Source: CAD feature listing. Evaluate the final solid. Frame: model axes, mm. Round coordinates to 2 decimals unless told otherwise and drop trailing zeros. Order: outer loops, then holes, each group sorted by start corner. A loop starts at its lowest first (then second) coordinate and runs counter-clockwise, first axis right, second up. Notation, with made-up numbers: (77.25, -13) - (127.25, -13) arc R25 ccw to (127.25, 6) - close; hole circle Ø1 at (10, 19.25). An arc over 180 degrees is marked (long way). Return JSON: item names as keys, results as strings. Group by question number.
1) Mould query, pull axis X, two halves, no side actions, for faces 1 (the cylindrical face through (79.297, -123.986, 1.521)), 2 (the cylindrical face through (-83, 99, 2)), 3 (the cylindrical face through (-43.67, 95.48, 1.48)). Classes: pulls with the +X half, pulls with the -X half, needs draft (parallel to the pull), parting line crosses it, or undercut.
2) Contact query for flat-ended pins moving along their axis: P1, Ø6, axis at x = 44, y = 93, coming from the +Z side; P2, Ø1, axis at x = -67.5, z = 1, coming from the -Y side. Output: stop coordinate, or through.
3) Section B-B, the plane x = -70. Return loops of the section in (y, z), plus the area to 3 significant figures.
4) Section A-A, the plane x = -44. Return loops of the section in (y, z).
5) Ray query, line 1 (Y direction, x = 11.5, z = 0.7); line 2 (Y direction, x = -44, z = 0.8); line 3 (Y direction, x = 77, z = 2.35). Return the intervals inside material, ascending. Write a range as from..to.
```python
from build123d import *

# Parameters (mm, degrees)
SKETCH_1_W          = 170
SKETCH_1_H          = 200
EXTRUDE_1_DEPTH     = 3
SKETCH_4_W          = 170
SKETCH_4_H          = 30
EXTRUDE_2_DEPTH     = 3
FILLET_1_R          = 20
FILLET_2_R          = 5
SKETCH_6_R          = 1.5
CUT_EXTRUDE_3_DEPTH = 4
SKETCH_7_R          = 2.5
CUT_EXTRUDE_4_DEPTH = 10


with BuildPart() as part:
    # 草图1 → 凸台-拉伸1 (new body)
    with BuildSketch(Plane.XY):
        Rectangle(SKETCH_1_W, SKETCH_1_H)
    extrude(amount=EXTRUDE_1_DEPTH)

    # 草图4 → 凸台-拉伸2 (add)
    with BuildSketch(Plane(origin=(0, 0, 0), x_dir=(-1, 0, 0), z_dir=(0, 0, -1))):
        with Locations((0, -115)):
            Rectangle(SKETCH_4_W, SKETCH_4_H)
    extrude(amount=-EXTRUDE_2_DEPTH)

    # 圆角1
    fillet_1_edges = [part.edges().sort_by_distance(p)[0] for p in [
        (-85, -130, 1.5),
        (85, -130, 1.5),
    ]]
    fillet(fillet_1_edges, radius=FILLET_1_R)

    # 圆角2
    fillet_2_edges = [part.edges().sort_by_distance(p)[0] for p in [
        (-85, 100, 1.5),
        (85, 100, 1.5),
    ]]
    fillet(fillet_2_edges, radius=FILLET_2_R)

    # 草图6 → 切除-拉伸3 (cut, through all)
    with BuildSketch(Plane.XY.offset(3)):
        with Locations((11.5, 5)):
            Circle(SKETCH_6_R)
        with Locations((11.5, 15)):
            Circle(SKETCH_6_R)
        with Locations((11.5, 65)):
            Circle(SKETCH_6_R)
        with Locations((11.5, 75)):
            Circle(SKETCH_6_R)
    extrude(amount=-CUT_EXTRUDE_3_DEPTH, mode=Mode.SUBTRACT)

    # 草图7 → 切除-拉伸4 (cut)
    with BuildSketch(Plane(origin=(0, 0, 0), x_dir=(-1, 0, 0), z_dir=(0, 0, -1))):
        with Locations((-18, 94.5)):
            Circle(SKETCH_7_R)
        with Locations((-70, 94.5)):
            Circle(SKETCH_7_R)
        with Locations((-44, 93)):
            Circle(SKETCH_7_R)
        with Locations((70, 94.5)):
            Circle(SKETCH_7_R)
        with Locations((44, 93)):
            Circle(SKETCH_7_R)
        with Locations((18, 94.5)):
            Circle(SKETCH_7_R)
    extrude(amount=-CUT_EXTRUDE_4_DEPTH, mode=Mode.SUBTRACT)


solid = part.part
```
Geometry check:
{
 "1": {"face 1": "pulls with the +X half", "face 2": "pulls with the -X half", "face 3": "undercut"},
 "2": {"P1": "z = 3", "P2": "y = -129.9"},
 "3": {"outline": "(-129.36, 0) - (92, 0) - (92, 3) - (-129.36, 3) - close; (97, 0) - (100, 0) - (100, 3) - (97, 3) - close", "area": "673 mm2"},
 "4": {"outline": "(-130, 0) - (90.5, 0) - (90.5, 3) - (-130, 3) - close; (95.5, 0) - (100, 0) - (100, 3) - (95.5, 3) - close"},
 "5": {"line 1": "-130..3.5, 6.5..13.5, 16.5..63.5, 66.5..73.5, 76.5..100", "line 2": "-130..90.5, 95.5..100", "line 3": "-126..100"}
}
